```python
from build123d import *

# Parameters (mm, degrees)
CUT_EXTRUDE1_DEPTH = 7


with BuildPart() as part:
    # Sketch1 → Revolve1 (revolve)
    with BuildSketch(Plane.XY):
        with BuildLine():
            Line((0, 0), (0, 15))
            ThreePointArc((0, 15), (2.888936029, 14.148226716), (5, 12))
            Line((5, 12), (5, 6))
            Line((5, 6), (4, 6))
            Line((4, 6), (4, 0))
            Line((4, 0), (0, 0))
        make_face()
    revolve(axis=Axis((0, 0, 0), (0, 1, 0)))

    # Sketch2 → Cut-Extrude1 (cut)
    with BuildSketch(Plane.XZ):
        Polygon((1.443375673, -2.5), (2.886751346, 0), (1.443375673, 2.5), (-1.443375673, 2.5), (-2.886751346, 0), (-1.443375673, -2.5), align=None)
    extrude(amount=-CUT_EXTRUDE1_DEPTH, mode=Mode.SUBTRACT)


solid = part.part
```
For this review, take the finished solid that the model builds, in its own axes (mm). Coordinates: 2 decimals unless noted, no trailing zeros. Order: outer loops, then holes, each group sorted by start corner. A loop starts at its lowest first (then second) coordinate and runs counter-clockwise, first axis right, second up. Notation, with made-up numbers: (73.25, 48.25) - (115.25, 48.25) arc R33 cw to (115.25, 83.25) - close; hole circle Ø7 at (-27, 79.25). An arc over 180 degrees is marked (long way). Answer as a JSON object with one key per item and string values. Group by question number.
1. We need section B-B on y = 7.25. State the section outline as (x, z) points, then the cut area to 3 significant figures.
2. We need section A-A on y = 2. State the section outline as (x, z) points.
3. Clearance check with flat-ended pins moving along their axes: P1, Ø1.4, axis at x = 0, y = 2.5, coming from the -Z side; P2, Ø3, axis at y = 13.5, z = 4, coming from the +X side; P3, Ø2.5, axis at x = -0.5, y = 3, coming from the +Z side. State where each tip first meets the part, or that it passes through.
4. For probe 1 along Z at (x, y) = (-2.75, 1.25); probe 2 along X at (y, z) = (0.5, -1.5); probe 3 along Z at (x, y) = (-1.75, 1), list the stretches that pass through material, from the lowest coordinate up.
5. The part is to be moulded in two halves that separate along Z. For faces 1 (the flat face through (0, 3, -2.5)), 2 (the flat face through (0, 0, 3)), 3 (the cylindrical face through (-1.08, 8.96, 4.88)), say which applies: pulls with the +Z half, pulls with the -Z half, needs draft (parallel to the pull), parting line crosses it, or undercut.
Final values:
{
 "1": {"outline": "circle Ø10 at (0, 0)", "area": "78.5 mm²"},
 "2": {"outline": "circle Ø8 at (0, 0); hole (-2.89, 0) - (-1.44, -2.5) - (1.44, -2.5) - (2.89, 0) - (1.44, 2.5) - (-1.44, 2.5) - close"},
 "3": {"P1": "z = -4", "P2": "x = 3.7", "P3": "z = 4"},
 "4": {"probe 1": "-2.9 to -0.24, 0.24 to 2.9", "probe 2": "-3.71 to -2.02, 2.02 to 3.71", "probe 3": "-3.6 to -1.97, 1.97 to 3.6"},
 "5": {"face 1": "undercut", "face 2": "needs draft", "face 3": "parting line crosses it"}
}
